```python
from build123d import *

# Parameters (mm, degrees)
BOSS_EXTRUDE1_DEPTH = 10
SKETCH2_R           = 4.010526774
SKETCH2_R_2         = 3.950911994
CUT_EXTRUDE2_DEPTH  = 10


with BuildPart() as part:
    # Sketch1 → Boss-Extrude1 (new body)
    with BuildSketch(Plane.XY):
        with BuildLine():
            ThreePointArc((-33.989040517, 36.142816718), (-67.185323929, -18.789245764), (-10.11434169, 10.577873726))
            ThreePointArc((-10.11434169, 10.577873726), (-18.277756389, 15.998303864), (-23.698186527, 7.834889164))
            ThreePointArc((-23.698186527, 7.834889164), (-57.057127067, -9.330681752), (-37.653346002, 22.778024532))
            ThreePointArc((-37.653346002, 22.778024532), (-29.138797167, 27.628267882), (-33.989040517, 36.142816718))
        make_face()
    extrude(amount=BOSS_EXTRUDE1_DEPTH)

    # Sketch2 → Cut-Extrude2 (cut)
    with BuildSketch(Plane.XY.offset(10)):
        with Locations((-35.907207797, 29.632235542)):
            Circle(SKETCH2_R)
        with Locations((-16.665002101, 9.172168726)):
            Circle(SKETCH2_R_2)
    extrude(amount=-CUT_EXTRUDE2_DEPTH, mode=Mode.SUBTRACT)


solid = part.part
```
The model under review builds one solid part; all positions refer to its coordinate system, in mm. Round coordinates to 2 decimals unless told otherwise and drop trailing zeros. Loops run counter-clockwise (first coordinate to the right, second up) from the corner with the lowest first, then second, coordinate; pieces in that order, holes last. Notation, with made-up numbers: (13, 77.5) - (63, 77.5) arc R7 ccw to (63, 88.5) - close; hole circle Ø9 at (-3, 19.5). An arc over 180 degrees is marked (long way). Write each question's results on one line, items separated by ' | '. Start each with the question number.
Q1. Draft analysis for pull direction Y (two halves, no side actions). For faces 1 (the cylindrical face through (-67.994, -17.891, 4.93)), 2 (the flat face through (-58, -10, 10)), 3 (the cylindrical face through (-38.9, 32.3, 5.1)), state which applies: pulls with the +Y half, pulls with the -Y half, needs draft (parallel to the pull), parting line crosses it, or undercut.
Q2. Take a section at C-C on z = 8. Give the boundary of the cut face in (x, y) (3 decimals).
Q3. Take a section at A-A on y = -11.5. Give the boundary of the cut face in (x, z), plus the area to 3 significant figures.
Q4. Insertion check: P1, Ø4, axis at x = -59, z = 5, coming from the -Y side; P2, Ø1.5, axis at y = 9.5, z = 3.5, coming from the -X side; P3, Ø2, axis at x = -57.5, z = 3, coming from the +Y side. Each pin has a flat end and moves straight along its axis. Give the tip position at first contact, or say it passes through.
Q5. Take a section at D-D on x = -65.5. Give the boundary of the cut face in (y, z), plus the area to 3 significant figures.
Q6. Wall thickness on line 1 along X through (y, z) = (8, 4.75); line 2 along Y through (x, z) = (-37.5, 3.25); line 3 along Y through (x, z) = (-36.5, 1.75): over which ranges is each line inside the solid? List them lowest first. Write a range as [from, to].
Q7. Take a section at B-B on x = -55.5. Give the boundary of the cut face in (y, z).
Data:
1) face 1: parting line crosses it | face 2: needs draft | face 3: undercut
2) outline: (-37.653, 22.778) arc R6.929 ccw to (-33.989, 36.143) arc R33.354 ccw (long way) to (-10.114, 10.578) arc R6.929 ccw to (-23.698, 7.835) arc R19.496 cw (long way) to start; hole circle Ø8.021 at (-35.907, 29.632); hole circle Ø7.902 at (-16.665, 9.172)
3) outline: (-72.35, 0) - (-54.67, 0) - (-54.67, 10) - (-72.35, 10) - close; (-30.95, 0) - (-13.26, 0) - (-13.26, 10) - (-30.95, 10) - close | area: 354 mm²
4) P1: stops at y = -26.21 | P2: stops at x = -75.82 | P3: stops at y = 34.39
5) outline: (-20.47, 0) - (28.42, 0) - (28.42, 10) - (-20.47, 10) - close | area: 489 mm²
6) line 1: x = [-75.92, -61.88], [-23.73, -20.44], [-12.89, -9.7] | line 2: y = [-28.95, -14.78], [22.74, 25.95], [33.31, 36.9] | line 3: y = [-28.78, -14.47], [22.56, 25.67], [33.6, 36.73]
7) outline: (-26.87, 0) - (-10.82, 0) - (-10.82, 10) - (-26.87, 10) - close; (18.78, 0) - (34.82, 0) - (34.82, 10) - (18.78, 10) - close
